from build123d import *

# Parameters (mm, degrees)
F1_DEPTH = 3
F2_R     = 1
F3_W     = 15.5
F3_H     = 3.5
F3_W_2   = 3.5
F3_H_2   = 15.5
F4_DEPTH = 25


with BuildPart() as f1:
    # F0 (on Front) → F1 (new body)
    with BuildSketch(Plane.XZ):
        with BuildLine():
            Line((0, 90), (0, 0))
            Line((0, 0), (110, 0))
            Line((110, 0), (110, 40.821911))
            Line((110, 40.821911), (105.5, 40.821911))
            Line((105.5, 40.821911), (105.5, 36.821911))
            ThreePointArc((105.5, 36.821911), (98, 29.321911), (90.5, 36.821911))
            Line((90.5, 36.821911), (90.5, 53.116433))
            Line((90.5, 53.116433), (86, 53.116433))
            Line((86, 53.116433), (86, 49.116433))
            ThreePointArc((86, 49.116433), (78.5, 41.616433), (71, 49.116433))
            Line((71, 49.116433), (71, 65.410955))
            Line((71, 65.410955), (66.5, 65.410955))
            Line((66.5, 65.410955), (66.5, 61.410955))
            ThreePointArc((66.5, 61.410955), (59, 53.910955), (51.5, 61.410955))
            Line((51.5, 61.410955), (51.5, 77.705478))
            Line((51.5, 77.705478), (47, 77.705478))
            Line((47, 77.705478), (47, 73.705478))
            ThreePointArc((47, 73.705478), (39.5, 66.205478), (32, 73.705478))
            Line((32, 73.705478), (32, 90))
            Line((32, 90), (27.5, 90))
            Line((27.5, 90), (27.5, 86))
            ThreePointArc((27.5, 86), (20, 78.5), (12.5, 86))
            Line((12.5, 86), (12.5, 90))
            Line((12.5, 90), (0, 90))
        make_face()
        with BuildLine():
            ThreePointArc((17, 12), (13.464466, 13.464466), (12, 17))
            Line((12, 17), (12, 61.883822))
            ThreePointArc((12, 61.883822), (14.584771, 66.261797), (19.666667, 66.113347))
            Line((19.666667, 66.113347), (90.855648, 21.229526))
            ThreePointArc((90.855648, 21.229526), (92.992502, 15.612129), (88.188981, 12))
            Line((88.188981, 12), (17, 12))
        make_face(mode=Mode.SUBTRACT)
    extrude(amount=F1_DEPTH)

    # F2
    f2_edges = [f1.edges().sort_by_distance(p)[0] for p in [
        (12.5, -1.5, 90),
        (27.5, -1.5, 90),
        (32, -1.5, 90),
        (47, -1.5, 77.705478),
        (51.5, -1.5, 77.705478),
        (66.5, -1.5, 65.410955),
        (71, -1.5, 65.410955),
        (110, -1.5, 40.821911),
        (105.5, -1.5, 40.821911),
        (90.5, -1.5, 53.116433),
        (86, -1.5, 53.116433),
    ]]
    fillet(f2_edges, radius=F2_R)

    # F3 (on face) → F4 (cut)
    with BuildSketch(Plane.XZ.offset(3)):
        with Locations((17.75, 5.75)):
            Rectangle(F3_W, F3_H)
        with Locations((92.75, 5.75)):
            Rectangle(F3_W, F3_H)
        with Locations((5.75, 17.75)):
            Rectangle(F3_W_2, F3_H_2)
        with Locations((5.75, 67.75)):
            Rectangle(F3_W_2, F3_H_2)
    extrude(amount=-F4_DEPTH, mode=Mode.SUBTRACT)


solid = f1.part
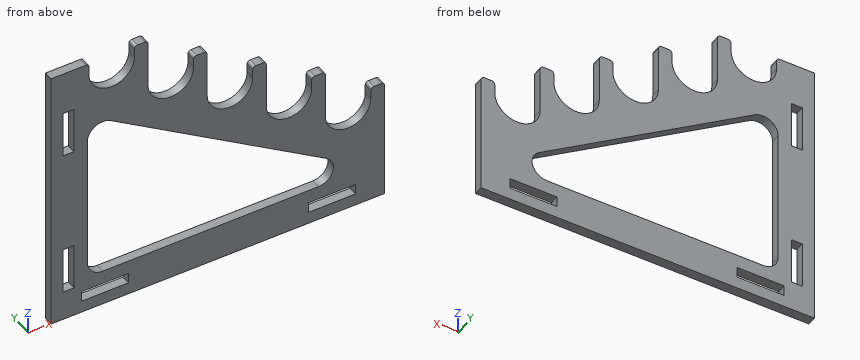
Work out the finished part from the listing and answer in its coordinate system (mm). Round coordinates to 2 decimals unless told otherwise and drop trailing zeros. Loops run counter-clockwise (first coordinate to the right, second up) from the corner with the lowest first, then second, coordinate; pieces in that order, holes last. Notation, with made-up numbers: (62, 19) - (90, 19) arc R8 cw to (90, 34) - close; hole circle Ø1 at (56.25, -37.5). An arc over 180 degrees is marked (long way). Use one line per item in the form item = value. Start each with the question number.
(1) Find section C-C on y = -1.7. Give the number of separate pieces and of enclosed holes in the cut face, and give its area (3 significant figures).
(2) Flat-ended cylindrical pins translate along their axes: P1, Ø1.5, axis at x = 94, y = -1.5, coming from the +Z side; P2, Ø1, axis at y = -2.5, z = 64, coming from the +X side; P3, Ø1.5, axis at x = 61.5, y = -2, coming from the +Z side. Find the tip coordinate at first contact, or state that the pin passes through.
(3) Find section D-D on x = 39.5. Determine the outline of the cut face in (y, z), and give its area (3 significant figures).
(4) Find section B-B on z = 47. Determine the outline of the cut face in (x, y), and give its area (3 significant figures).
(5) Find section A-A on x = 53. Determine the outline of the cut face in (y, z).
(6) Consider line 1 (Z direction, x = 87, y = -1); line 2 (X direction, y = -2.25, z = 20.5); line 3 (Z direction, x = 13.5, y = -2.1). Determine where each line is inside the solid, lowest interval first.
Answer list:
q1.separate_pieces = 1
q1.enclosed_holes = 5
q1.area = 3,860 mm^2
q2.P1 = 31.02
q2.P2 = 71
q2.P3 = 54.65
q3.outline = (-3, 0) - (0, 0) - (0, 12) - (-3, 12) - close; (-3, 53.61) - (0, 53.61) - (0, 66.21) - (-3, 66.21) - close
q3.area = 73.8 mm^2
q4.outline = (0, -3) - (12, -3) - (12, 0) - (0, 0) - close; (49.98, -3) - (71.3, -3) - (71.3, 0) - (49.98, 0) - close; (85.7, -3) - (90.5, -3) - (90.5, 0) - (85.7, 0) - close
q4.area = 114 mm^2
q5.outline = (-3, 0) - (0, 0) - (0, 12) - (-3, 12) - close; (-3, 45.1) - (0, 45.1) - (0, 56.91) - (-3, 56.91) - close
q6.line_1 = 0 to 4, 7.5 to 12, 23.66 to 53.12
q6.line_2 = 0 to 4, 7.5 to 12, 91.76 to 110
q6.line_3 = 0 to 4, 7.5 to 13.43, 65.45 to 82.26
